The drawing under review shows one solid part. Ordinate dimensions are in mm from its lowest x, y, z. A direction names the side the tool comes from. Coordinates: 2 decimals unless noted, no trailing zeros. Write each loop counter-clockwise with the first axis right and the second up, starting at its lowest first coordinate (ties: lowest second). Pieces come first, ordered by that corner, then holes. Notation, with made-up numbers: M 3.5,51 L 56.5,51 A12 ccw 56.5,65 Z; hole C 80,35.5 d10. An arc over 180 degrees is marked long. Answer as CSV lines item,"result". Start each with the question number.
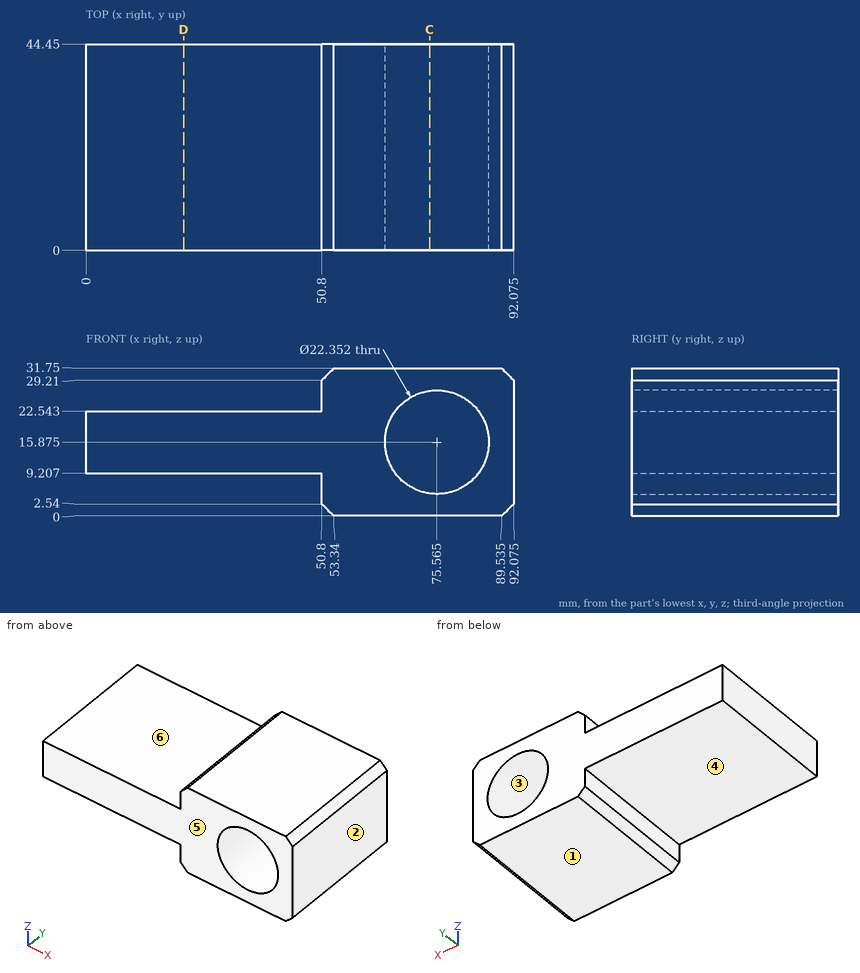
1) Take a section at D-D on x = 21. Give the boundary of the cut face in (y, z).
2) Clearance check with flat-ended pins moving along their axes: pin 1 Ø22 at (x, y) = (25, 12.5) entering from +Z; pin 2 Ø5 at (y, z) = (11.5, 25.5) entering from -X; pin 3 Ø2 at (x, y) = (16, 19.5) entering from -Z; pin 4 Ø18 at (x, z) = (75.565, 15.875) entering from +Y. State where each tip first meets the part, or that it passes through.
3) To check wall thickness, follow line 1 (X direction, y = 13, z = 9) (1 decimal); line 2 (X direction, y = 31.5, z = 20.5) (1 decimal); line 3 (Z direction, x = 42, y = 30.5). State the ranges of each line that lie inside material, in increasing order. Write a range as [from, to].
4) Take a section at C-C on x = 74. Give the boundary of the cut face in (y, z).
5) Tool access review of the marked faces 4, 5 and 6: name each direction out of +Z, -Z, +X, -X, +Y, -Y from which nothing blocks a thin tool from reaching the whole face with its end or side.
6) Mouldability with a two-part tool opening along X and no side actions: class the marked faces 1, 2 and 3 as +X half, -X half, draft (parallel to the pull), parting line (faces both ways), or undercut.
Results:
1,outline,"M 0,9.21 L 44.45,9.21 L 44.45,22.54 L 0,22.54 Z"
2,pin 1,"stops at z = 22.54"
2,pin 2,"stops at x = 50.8"
2,pin 3,"stops at z = 9.21"
2,pin 4,"passes through"
3,line 1,"x = [50.8, 66.8], [84.4, 92.1]"
3,line 2,"x = [0, 65.4], [85.7, 92.1]"
3,line 3,"z = [9.21, 22.54]"
4,outline,"M 0,0 L 44.45,0 L 44.45,4.81 L 0,4.81 Z; M 0,26.94 L 44.45,26.94 L 44.45,31.75 L 0,31.75 Z"
5,face 4,"-Z, -X, +Y, -Y"
5,face 5,"+Z, -Z, +X, -X, -Y"
5,face 6,"+Z, -X, +Y, -Y"
6,face 1,"draft"
6,face 2,"+X half"
6,face 3,"undercut"
